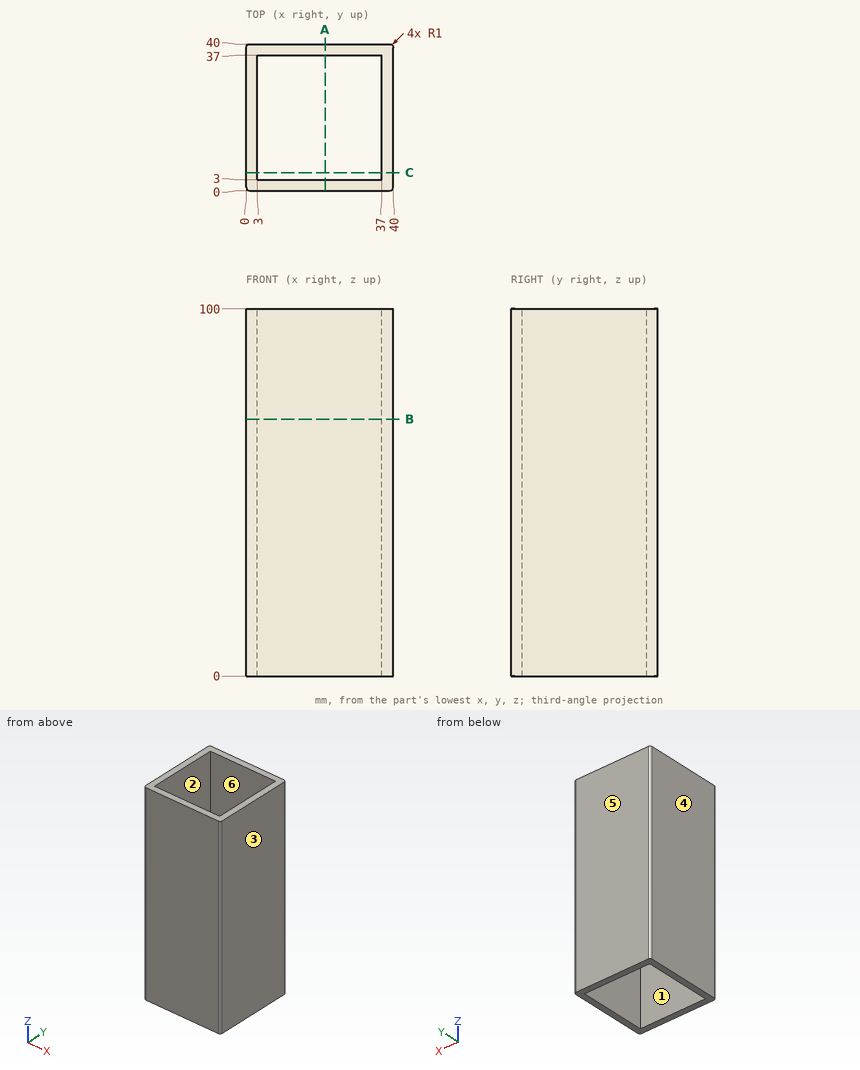
For this review, use the dimensioned drawing (mm, ordinates from the lowest corner) and the shaded views. A direction names the side the tool comes from. Round coordinates to 2 decimals unless told otherwise and drop trailing zeros. Write each loop counter-clockwise with the first axis right and the second up, starting at its lowest first coordinate (ties: lowest second). Pieces come first, ordered by that corner, then holes. Notation, with made-up numbers: (43.5, 45.5) - (81.5, 45.5) arc R17 cw to (81.5, 62.5) - close; hole circle Ø1 at (63, 46). An arc over 180 degrees is marked (long way). Use a Markdown table: item, result.
Q1. We need section A-A (x = 21.5). Give the boundary of the cut face in (y, z), plus the area to 3 significant figures.
Derived:
| item | result |
|---|---|
| outline | (0, 0) - (3, 0) - (3, 100) - (0, 100) - close; (37, 0) - (40, 0) - (40, 100) - (37, 100) - close |
| area | 600 mm2 |
Q2. We need section B-B (z = 70). Give the boundary of the cut face in (x, y), plus the area to 3 significant figures.
Derived:
| item | result |
|---|---|
| outline | (0, 1) arc R1 ccw to (1, 0) - (39, 0) arc R1 ccw to (40, 1) - (40, 39) arc R1 ccw to (39, 40) - (1, 40) arc R1 ccw to (0, 39) - close; hole (3, 3) - (37, 3) - (37, 37) - (3, 37) - close |
| area | 443 mm2 |
Q3. Machinability: for the marked faces 5 and 6, which of the approach directions +Z, -Z, +X, -X, +Y, -Y give a long, thin tool a straight path to every point of the face, cutting with its end or side? Answer none if there is none.
Derived:
| item | result |
|---|---|
| face 5 | +Z, -Z, +X, -X, +Y |
| face 6 | +Z, -Z |
Q4. The part is to be moulded in two halves that separate along X. For the marked faces 1, 2, 3 and 4, say which applies: pulls with the +X half, pulls with the -X half, needs draft (parallel to the pull), parting line crosses it, or undercut.
Derived:
| item | result |
|---|---|
| face 1 | undercut |
| face 2 | undercut |
| face 3 | pulls with the +X half |
| face 4 | pulls with the -X half |
Q5. Wall thickness on line 1 along X through (y, z) = (7.5, 5): over which ranges is the line inside the solid? List them lowest first.
Derived:
| item | result |
|---|---|
| line 1 | x = 0 to 3, 37 to 40 |
Q6. Clearance check with a flat-ended pin moving along its axis: pin 1 (10 mm diameter, centred on y = 7.5, z = 78.5, fed in from -X). State where the tip first meets the part, or that it passes through.
Derived:
| item | result |
|---|---|
| pin 1 | stops at x = 0 |
